from build123d import *

# Parameters (mm, degrees)
SKETCH1_W          = 52.8624
SKETCH1_H          = 22.352
BASE_FLANGE1_DEPTH = 3.175
SKETCH6_R          = 4.445
CUT_EXTRUDE1_DEPTH = 3.175
FILLET1_R          = 6.35


# Sheet-metal steps are written as plain solids
with BuildPart() as part:
    # Sketch1 → Base-Flange1 (new body)
    with BuildSketch(Plane.XY):
        with Locations((26.4312, 11.176)):
            Rectangle(SKETCH1_W, SKETCH1_H)
    extrude(amount=-BASE_FLANGE1_DEPTH)

    # Sketch6 → Cut-Extrude1 (cut)
    with BuildSketch(Plane.XY):
        with Locations((9.525, 11.176)):
            Circle(SKETCH6_R)
        with BuildLine():
            Line((42.9437, 6.8072), (43.7311, 6.8072))
            ThreePointArc((43.7311, 6.8072), (48.0999, 11.176), (43.7311, 15.5448))
            Line((43.7311, 15.5448), (42.9437, 15.5448))
            ThreePointArc((42.9437, 15.5448), (38.5749, 11.176), (42.9437, 6.8072))
        make_face()
    extrude(amount=-CUT_EXTRUDE1_DEPTH, mode=Mode.SUBTRACT)

    # Fillet1
    fillet1_edges = [part.edges().sort_by_distance(p)[0] for p in [
        (0, 22.352, -1.5875),
        (52.8624, 22.352, -1.5875),
        (52.8624, 0, -1.5875),
        (0, 0, -1.5875),
    ]]
    fillet(fillet1_edges, radius=FILLET1_R)


solid = part.part
Could you check a few things on this model? Use its own coordinates, in mm. A direction names the side the tool comes from. Give positions to 0.01 mm unless a question says otherwise; leave off trailing zeros. Order: outer loops, then holes, each group sorted by start corner. A loop starts at its lowest first (then second) coordinate and runs counter-clockwise, first axis right, second up. Notation, with made-up numbers: (-3, 25.25) - (46, 25.25) arc R28 ccw to (46, 57.25) - close; hole circle Ø1 at (-38.5, 73). An arc over 180 degrees is marked (long way). Return JSON: item names as keys, results as strings. Group by question number.
Q1. Suppose I cut it at C-C, the plane z = -2.1. Please give me the cut outline in (x, y) (3 decimals).
Q2. Thinking about a two-plate mould opening in X: for faces 3 (the face through (1.81, 20.44, -1.61)), 4 (the face through (26, 22.352, -2)), 5 (the face through (38.576, 11.272, -1.565)), 6 (the face through (50.95, 1.81, -1.61)), which applies, pulls with the +X half, pulls with the -X half, needs draft (parallel to the pull), parting line crosses it, or undercut?
Q3. Will this pin go through, and if not, where does the flat tip stop? pin 1 Ø8 at (x, y) = (9.525, 11.176) entering from +Z.
Q4. Suppose I cut it at A-A, the plane y = 14.75. Please give me the cut outline in (x, z) (3 decimals), and give its area (3 significant figures).
Q5. Suppose I cut it at D-D, the plane y = 8. Please give me the cut outline in (x, z) (3 decimals).
Q6. Please list where these lines run through material, in increasing order: line 1 along X through (y, z) = (11.25, -1.45); line 2 along X through (y, z) = (9.25, -1.55); line 3 along Y through (x, z) = (13, -1.4). Write a range as [from, to].
Q7. Which directions (+Z, -Z, +X, -X, +Y, -Y) give clear straight access to the entire face, cutting with the end or side of a thin tool? Please do faces 1 (the face through (0, 11, -2)), 2 (the face through (48.1, 11.1, -1.6)).
Q8. Suppose I cut it at B-B, the plane x = 39.5. Please give me the cut outline in (y, z) (3 decimals).
Resolved:
{
 "1": {"outline": "(0, 6.35) arc R6.35 ccw to (6.35, 0) - (46.512, 0) arc R6.35 ccw to (52.862, 6.35) - (52.862, 16.002) arc R6.35 ccw to (46.512, 22.352) - (6.35, 22.352) arc R6.35 ccw to (0, 16.002) - close; hole circle Ø8.89 at (9.525, 11.176); hole (42.944, 6.807) - (43.731, 6.807) arc R4.369 ccw to (43.731, 15.545) - (42.944, 15.545) arc R4.369 ccw to start"},
 "2": {"face 3": "pulls with the -X half", "face 4": "needs draft", "face 5": "undercut", "face 6": "pulls with the +X half"},
 "3": {"pin 1": "passes through"},
 "4": {"outline": "(0, -3.175) - (6.882, -3.175) - (6.882, 0) - (0, 0) - close; (12.168, -3.175) - (40.431, -3.175) - (40.431, 0) - (12.168, 0) - close; (46.244, -3.175) - (52.862, -3.175) - (52.862, 0) - (46.244, 0) - close", "area": "133 mm2"},
 "5": {"outline": "(0, -3.175) - (6.415, -3.175) - (6.415, 0) - (0, 0) - close; (12.635, -3.175) - (39.944, -3.175) - (39.944, 0) - (12.635, 0) - close; (46.731, -3.175) - (52.862, -3.175) - (52.862, 0) - (46.731, 0) - close"},
 "6": {"line 1": "x = [0, 5.08], [13.97, 38.58], [48.1, 52.86]", "line 2": "x = [0, 5.52], [13.53, 39.02], [47.65, 52.86]", "line 3": "y = [0, 8.4], [13.95, 22.35]"},
 "7": {"face 1": "+Z, -Z, -X, +Y, -Y", "face 2": "+Z, -Z"},
 "8": {"outline": "(0, -3.175) - (8.488, -3.175) - (8.488, 0) - (0, 0) - close; (13.864, -3.175) - (22.352, -3.175) - (22.352, 0) - (13.864, 0) - close"}
}
